Could you check a few things on this model? Use its own coordinates, in mm. A direction names the side the tool comes from. Coordinates: 2 decimals unless noted, no trailing zeros. Write each loop counter-clockwise with the first axis right and the second up, starting at its lowest first coordinate (ties: lowest second). Pieces come first, ordered by that corner, then holes. Notation, with made-up numbers: M 35.5,-32 L 46.5,-32 A8 ccw 46.5,-23 Z; hole C 1.25,67.5 d6. An arc over 180 degrees is marked long. Write item = value, one per line.
```python
from build123d import *

# Parameters (mm, degrees)
BOSS_EXTRUDE1_DEPTH = 12.7
SKETCH5_R           = 1.5875
CUT_EXTRUDE1_DEPTH  = 5.7625
SKETCH6_R           = 1.5875
CUT_EXTRUDE2_DEPTH  = 5.7625


with BuildPart() as part:
    # Sketch1 → Boss-Extrude1 (new body)
    with BuildSketch(Plane(origin=(0, 0, 0), x_dir=(1, 0, 0), z_dir=(0, 1, 0))):
        with BuildLine():
            Line((-55.5625, 0), (-84.1375, 0))
            Line((-84.1375, 0), (-84.1375, 12.7))
            Line((-84.1375, 12.7), (-79.375, 12.7))
            Line((-79.375, 12.7), (-79.375, 4.7625))
            Line((-79.375, 4.7625), (-60.136712736, 4.7625))
            ThreePointArc((-60.136712736, 4.7625), (0, 60.325), (60.136712736, 4.7625))
            Line((60.136712736, 4.7625), (79.375, 4.7625))
            Line((79.375, 4.7625), (79.375, 12.7))
            Line((79.375, 12.7), (84.1375, 12.7))
            Line((84.1375, 12.7), (84.1375, 0))
            Line((84.1375, 0), (55.5625, 0))
            ThreePointArc((55.5625, 0), (0, 55.5625), (-55.5625, 0))
        make_face()
    extrude(amount=BOSS_EXTRUDE1_DEPTH)

    # Sketch5 → Cut-Extrude1 (cut, through all)
    with BuildSketch(Plane(origin=(0, 0, -4.7625), x_dir=(-1, 0, 0), z_dir=(0, 0, -1))):
        with Locations((69.755856368, 6.35)):
            Circle(SKETCH5_R)
    cut_extrude1 = extrude(amount=-CUT_EXTRUDE1_DEPTH, mode=Mode.SUBTRACT)

    # Sketch6 → Cut-Extrude2 (cut, through all)
    with BuildSketch(Plane(origin=(-79.375, 0, 0), x_dir=(0, 0, -1), z_dir=(1, 0, 0))):
        with Locations((8.73125, 6.35)):
            Circle(SKETCH6_R)
    cut_extrude2 = extrude(amount=-CUT_EXTRUDE2_DEPTH, mode=Mode.SUBTRACT)

    # Mirror2: Cut-Extrude1, Cut-Extrude2 across plane
    add(cut_extrude1.mirror(Plane(origin=(0, 0, 0), x_dir=(0, 0, 1), z_dir=(1, 0, 0))), mode=Mode.SUBTRACT)
    add(cut_extrude2.mirror(Plane(origin=(0, 0, 0), x_dir=(0, 0, 1), z_dir=(1, 0, 0))), mode=Mode.SUBTRACT)


solid = part.part
```
Item 1: Imagine slicing it at A-A (y = 6.35). State how many separate pieces and enclosed holes the cut face has, and give its area (3 significant figures).
Numbers:
separate_pieces = 5
enclosed_holes = 0
area = 1,110 mm²
Item 2: I'm going to push flat-ended pins straight in: P1, Ø4, axis at y = 7, z = -26, coming from the -X side; P2, Ø6.5, axis at x = 69, y = 3.5, coming from the -Z side; P3, Ø1.9, axis at y = 6.35, z = -8.73, coming from the +X side; P4, Ø4, axis at x = -69.76, y = 6.35, coming from the +Z side. Where does each tip first touch, or does it pass through?
Numbers:
P1 = -55.35
P2 = -4.76
P3 = 59.82
P4 = 0
Item 3: For faces 4 (the face through (-82, 6, -12.7)), 5 (the face through (-79.375, 5, -10)), 6 (the face through (82, 6, -12.7)), 7 (the face through (81.723, 5.742, -10.198)), which set-ups out of +Z, -Z, +X, -X, +Y, -Y let a thin tool reach every point of the face, with its end or its side?
Numbers:
face_4 = -Z, -X, +Y, -Y
face_5 = -Z, +Y, -Y
face_6 = -Z, +X, +Y, -Y
face_7 = +X
Item 4: Imagine slicing it at B-B (z = -35). Write out the boundary of the cut face in (x, y), and give its area (3 significant figures).
Numbers:
outline = M -49.13,0 L -43.15,0 L -43.15,12.7 L -49.13,12.7 Z; M 43.15,0 L 49.13,0 L 49.13,12.7 L 43.15,12.7 Z
area = 152 mm²
Item 5: Imagine slicing it at D-D (z = -51.5). Write out the boundary of the cut face in (x, y), and give its area (3 significant figures).
Numbers:
outline = M -31.41,0 L -20.86,0 L -20.86,12.7 L -31.41,12.7 Z; M 20.86,0 L 31.41,0 L 31.41,12.7 L 20.86,12.7 Z
area = 268 mm²
Item 6: Imagine slicing it at C-C (x = 0). Write out the boundary of the cut face in (y, z) (1 decimal), and give its area (3 significant figures).
Numbers:
outline = M 0,-60.3 L 12.7,-60.3 L 12.7,-55.6 L 0,-55.6 Z
area = 60.5 mm²
Item 7: If I drill on line 1 along Z through (x, y) = (82.6, 6.35); line 2 along X through (y, z) = (0.5, -11) (1 decimal); line 3 along X through (y, z) = (6.5, -5) (1 decimal), over which ranges is the centre line in solid material (lowest first)?
Numbers:
line_1 = -12.7 to -10.32, -7.14 to 0
line_2 = -84.1 to -79.4, -59.3 to -54.5, 54.5 to 59.3, 79.4 to 84.1
line_3 = -84.1 to -79.4, -60.1 to -55.3, 55.3 to 60.1, 79.4 to 84.1
Item 8: If we mould it in two halves opening along Y, with no side actions, what happens to faces 1 (the face through (-81.723, 5.742, -10.198)), 2 (the face through (0, 12.7, -57)), 3 (the face through (-68, 6, -4.762))? For each: pulls with the +Y half, pulls with the -Y half, needs draft (parallel to the pull), parting line crosses it, or undercut.
Numbers:
face_1 = undercut
face_2 = pulls with the +Y half
face_3 = needs draft
